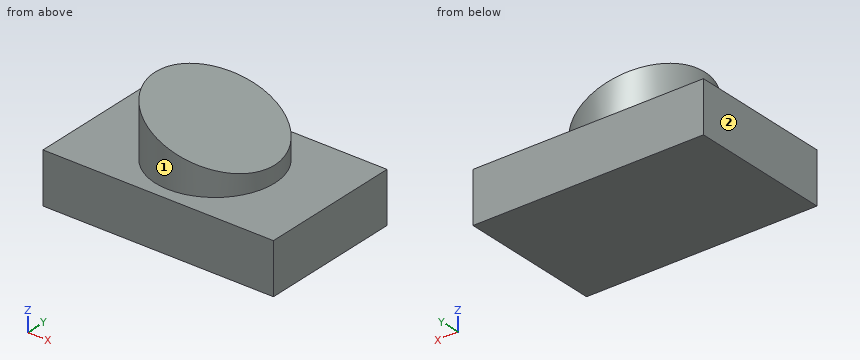
```python
from build123d import *

# Parameters (mm, degrees)
F0_W     = 122.473546
F0_H     = 26.955904
F1_DEPTH = 76.2
F2_R     = 31.75
F3_DEPTH = 38.1
F5_DEPTH = 92.71


with BuildPart() as f1:
    # F0 (on Front) → F1 (new body)
    with BuildSketch(Plane.XZ):
        Rectangle(F0_W, F0_H)
    extrude(amount=F1_DEPTH)

    # F2 (on face) → F3 (join)
    with BuildSketch(Plane.XY.offset(13.477952)):
        with Locations((0, -38.1)):
            Circle(F2_R)
    extrude(amount=F3_DEPTH)

    # F4 (on Front) → F5 (cut)
    with BuildSketch(Plane.XZ):
        Polygon((38.983259, 69.250525), (-120.331847, 75.206235), (38.983259, 19.648822), align=None)
    extrude(amount=F5_DEPTH, mode=Mode.SUBTRACT)


solid = f1.part
```
Geometry check sheet. Reference: the model listing, model coordinates, mm. Face numbers are marked on the shaded views. A direction names the side the tool comes from. Give positions to 0.01 mm unless a question says otherwise; leave off trailing zeros. Write each loop counter-clockwise with the first axis right and the second up, starting at its lowest first coordinate (ties: lowest second). Pieces come first, ordered by that corner, then holes. Notation, with made-up numbers: (73, 0) -> (105, 0) arc R19 cw to (105, 32) -> close; hole circle Ø3 at (-4.5, 43). An arc over 180 degrees is marked (long way). Use one line per item in the form item = value.
Item 1: Sectioned sample at B-B on x = 0. Enter the section's corners in (y, z).
Results list:
outline = (-76.2, -13.48) -> (0, -13.48) -> (0, 13.48) -> (-6.35, 13.48) -> (-6.35, 33.24) -> (-69.85, 33.24) -> (-69.85, 13.48) -> (-76.2, 13.48) -> close
Item 2: Depth check by flat-ended pin: pin 1 Ø5 at (x, y) = (-16.5, -9.5) entering from +Z; pin 2 Ø1.5 at (x, y) = (-46.5, -49) entering from +Z; pin 3 Ø10 at (x, z) = (3, 20.5) entering from -Y. Enter the tip coordinate at first touch or a pass-through.
Results list:
pin_1 = 39.4
pin_2 = 13.48
pin_3 = -69.85
Item 3: Sectioned sample at D-D on y = -4.5. Enter the section's corners in (x, z), plus the area to 3 significant figures.
Results list:
outline = (-61.24, -13.48) -> (61.24, -13.48) -> (61.24, 13.48) -> (-61.24, 13.48) -> close
area = 3,300 mm2
Item 4: Scan lines: line 1 (Z direction, x = 42, y = -35); line 2 (Y direction, x = 0, z = 17); line 3 (Z direction, x = -6.5, y = -61.5). Record each from-to range of solid material in increasing order.
Results list:
line_1 = -13.48 to 13.48
line_2 = -69.85 to -6.35
line_3 = -13.48 to 35.51
Item 5: Sectioned sample at A-A on y = -38.1. Enter the section's corners in (x, z).
Results list:
outline = (-61.24, -13.48) -> (61.24, -13.48) -> (61.24, 13.48) -> (31.75, 13.48) -> (31.75, 22.17) -> (-31.75, 44.32) -> (-31.75, 13.48) -> (-61.24, 13.48) -> close
Item 6: Sectioned sample at C-C on x = 37. Enter the section's corners in (y, z).
Results list:
outline = (-76.2, -13.48) -> (0, -13.48) -> (0, 13.48) -> (-76.2, 13.48) -> close
Item 7: Access from +Z, -Z, +X, -X, +Y, -Y to the whole of each face (thin tool, end or side, straight path). Record for the marked faces 1 and 2.
Results list:
face_1 = +Z
face_2 = +Z, -Z, -X, +Y, -Y
